Check sheet for the modelled part. Datum: model origin and axes. Units: mm. Face numbers are marked on the shaded views. Coordinates: 2 decimals unless noted, no trailing zeros. Loops run counter-clockwise (first coordinate to the right, second up) from the corner with the lowest first, then second, coordinate; pieces in that order, holes last. Notation, with made-up numbers: M 32.5,38.25 L 36.5,38.25 A23 ccw 36.5,65.25 Z; hole C -19,56 d6. An arc over 180 degrees is marked long. Answer as CSV lines item,"result". Start each with the question number.
from build123d import *

# Parameters (mm, degrees)
F1_DEPTH = 9.525
F3_DEPTH = 50.8
F5_DEPTH = 50.8


with BuildPart() as f1:
    # F0 (on Top) → F1 (new body)
    with BuildSketch(Plane.XY):
        with BuildLine():
            ThreePointArc((-88.9, 0), (0, 88.9), (88.9, 0))
            ThreePointArc((88.9, 0), (96.339488, -17.960512), (114.3, -25.4))
            Line((114.3, -25.4), (152.717048, -25.4))
            Line((152.717048, -25.4), (152.717048, 25.4))
            Line((152.717048, 25.4), (111.442048, 25.4))
            ThreePointArc((111.442048, 25.4), (0, 114.3), (-111.442048, 25.4))
            Line((-111.442048, 25.4), (-152.717048, 25.4))
            Line((-152.717048, 25.4), (-152.717048, -25.4))
            Line((-152.717048, -25.4), (-114.3, -25.4))
            ThreePointArc((-114.3, -25.4), (-96.339488, -17.960512), (-88.9, 0))
        make_face()
    extrude(amount=F1_DEPTH)

    # F2 (on face) → F3 (join, through all)
    with BuildSketch(Plane.XZ.offset(25.4)):
        Polygon((161.697304, 0.544744), (152.717048, 9.525), (148.771664, 0), (154.962112, -6.190448), align=None)
    extrude(amount=-F3_DEPTH)

    # F4 (on face) → F5 (join, through all)
    with BuildSketch(Plane.XZ.offset(25.4)):
        Polygon((-148.771664, 0), (-152.717048, 9.525), (-161.697304, 0.544744), (-154.962112, -6.190448), align=None)
    extrude(amount=-F5_DEPTH)


solid = f1.part
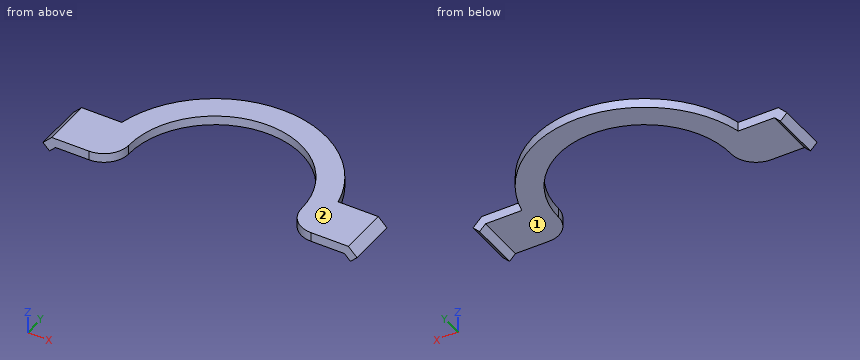
Item 1: Sectioned sample at A-A, the plane y = 80. Record the boundary of the cut face in (x, z) (3 decimals).
Item 2: Sectioned sample at D-D, the plane x = -125. Record the boundary of the cut face in (y, z) (3 decimals).
Item 3: Sectioned sample at C-C, the plane y = 46. Record the boundary of the cut face in (x, z) (3 decimals).
Item 4: Go/stop test with flat-tipped pins: pin 1 (1 mm diameter, centred on x = 111, z = 2, fed in from -Y); pin 2 (4 mm diameter, centred on x = 85, y = 47.5, fed in from -Z); pin 3 (8 mm diameter, centred on x = -35, z = -1.5, fed in from -Y). Record where each tip stops, or that it passes through.
Item 5: Material ranges on line 1 (Y direction, x = -148, z = 6.75); line 2 (Z direction, x = 18, y = 97) (3 decimals); line 3 (X direction, y = 37, z = 7.5), recorded low to high. Write a range as from..to.
Item 6: Sectioned sample at B-B, the plane z = 4.5. Record the boundary of the cut face in (x, y), and give its area (3 significant figures).
Item 7: Release check for a two-part mould opening along X. For the marked faces 1 and 2 record: released by +X, released by -X, zero draft, split by the parting line, or undercut.
Reply:
1,outline,"M -81.636,0 L -38.771,0 L -38.771,9.525 L -81.636,9.525 Z; M 38.771,0 L 81.636,0 L 81.636,9.525 L 38.771,9.525 Z"
2,outline,"M -25.4,0 L 25.4,0 L 25.4,9.525 L -25.4,9.525 Z"
3,outline,"M -104.635,0 L -76.074,0 L -76.074,9.525 L -104.635,9.525 Z; M 76.074,0 L 104.635,0 L 104.635,9.525 L 76.074,9.525 Z"
4,pin 1,"y = -25.25"
4,pin 2,"z = 0"
4,pin 3,"y = 80.03"
5,line 1,"-25.4..25.4"
5,line 2,"0..9.525"
5,line 3,"-108.15..-80.83, 80.83..108.15"
6,outline,"M -157.74,-25.4 L -114.3,-25.4 A25.4 ccw -88.9,0 A88.9 cw 88.9,0 A25.4 ccw 114.3,-25.4 L 157.74,-25.4 L 157.74,25.4 L 111.44,25.4 A114.3 ccw -111.44,25.4 L -157.74,25.4 Z"
6,area,"13,600 mm²"
7,face 1,"undercut"
7,face 2,"zero draft"
